from build123d import *

# Parameters (mm, degrees)
SKETCH1_W           = 66.8
SKETCH1_H           = 14
SKETCH1_R           = 1.1
BOSS_EXTRUDE2_DEPTH = 7
SKETCH5_W           = 66.8
SKETCH5_H           = 1.5
BOSS_EXTRUDE3_DEPTH = 93
SKETCH6_W           = 66.8
SKETCH6_H           = 93
SKETCH6_R           = 1
SKETCH6_W_2         = 60.8
SKETCH6_H_2         = 87
BOSS_EXTRUDE4_DEPTH = 10
FILLET1_R           = 1
CUT_EXTRUDE1_DEPTH  = 10


with BuildPart() as part:
    # Sketch1 → Boss-Extrude2 (new body)
    with BuildSketch(Plane.XY):
        Rectangle(SKETCH1_W, SKETCH1_H)
        Circle(SKETCH1_R, mode=Mode.SUBTRACT)
    extrude(amount=BOSS_EXTRUDE2_DEPTH)

    # Sketch5 → Boss-Extrude3 (add)
    with BuildSketch(Plane.XY.offset(7)):
        with Locations((0, -6.25)):
            Rectangle(SKETCH5_W, SKETCH5_H)
    extrude(amount=BOSS_EXTRUDE3_DEPTH)

    # Sketch6 → Boss-Extrude4 (add)
    with BuildSketch(Plane(origin=(0, -5.5, 0), x_dir=(1, 0, 0), z_dir=(0, 1, 0))):
        with Locations((0, -53.5)):
            Rectangle(SKETCH6_W, SKETCH6_H)
        with Locations(Location((-31.45, -8.95, 0), (0, 0, 270))):
            Circle(SKETCH6_R, mode=Mode.SUBTRACT)
        with Locations(Location((31.45, -8.95, 0), (0, 0, 270))):
            Circle(SKETCH6_R, mode=Mode.SUBTRACT)
        with Locations(Location((31.45, -98.05, 0), (0, 0, 270))):
            Circle(SKETCH6_R, mode=Mode.SUBTRACT)
        with Locations(Location((-31.45, -98.05, 0), (0, 0, 270))):
            Circle(SKETCH6_R, mode=Mode.SUBTRACT)
        with Locations((0, -53.5)):
            Rectangle(SKETCH6_W_2, SKETCH6_H_2, mode=Mode.SUBTRACT)
    extrude(amount=BOSS_EXTRUDE4_DEPTH)

    # Fillet1
    fillet1_edges = [part.edges().sort_by_distance(p)[0] for p in [
        (30.4, -0.5, 97),
        (30.4, -0.5, 10),
        (-30.4, -0.5, 10),
        (-30.4, -0.5, 97),
    ]]
    fillet(fillet1_edges, radius=FILLET1_R)

    # Sketch2 → Cut-Extrude1 (cut)
    with BuildSketch(Plane(origin=(0, 0, 0), x_dir=(-1, 0, 0), z_dir=(0, 0, -1))):
        with BuildLine():
            Line((2.7, 0), (4.75, 0))
            ThreePointArc((4.75, 0), (1.723006094, -4.426482802), (-3.5, -3.211308145))
            Line((-3.5, -3.211308145), (-1.989473684, -1.825375156))
            ThreePointArc((-1.989473684, -1.825375156), (0.979392938, -2.516106014), (2.7, 0))
        make_face()
    extrude(amount=-CUT_EXTRUDE1_DEPTH, mode=Mode.SUBTRACT)


solid = part.part
Model file for the job. Use its own axes, mm. A direction names the side the tool comes from. Give positions to 0.01 mm unless a question says otherwise; leave off trailing zeros. Order: outer loops, then holes, each group sorted by start corner. A loop starts at its lowest first (then second) coordinate and runs counter-clockwise, first axis right, second up. Notation, with made-up numbers: (19.5, -37.75) - (78.5, -37.75) arc R35 ccw to (78.5, 0.25) - close; hole circle Ø10 at (-30, -30). An arc over 180 degrees is marked (long way). Return JSON: item names as keys, results as strings.
1) Pull direction Z, two halves, no side cores. Call faces 1 (the flat face through (0, 2, 0)), 2 (the flat face through (-33.4, -2, 51)), 3 (the flat face through (0, -1, 10)): pulls with the +Z half, pulls with the -Z half, needs draft (parallel to the pull), parting line crosses it, or undercut.
Geometry says:
{"face 1": "pulls with the -Z half", "face 2": "needs draft", "face 3": "undercut"}
2) Cut at D-D, the plane z = 28.5. Give the cut face in (x, y).
Geometry says:
{"outline": "(-33.4, -7) - (33.4, -7) - (33.4, 4.5) - (30.4, 4.5) - (30.4, -5.5) - (-30.4, -5.5) - (-30.4, 4.5) - (-33.4, 4.5) - close"}
3) 3-axis set-ups, long thin cutter, end or side, ignore diameter. For faces 4 (the flat face through (31, -5.5, 98)), 5 (the flat face through (-32, 4.5, 50)), 6 (the cylindrical face through (-1.797, -4.397, 4.93)): which of +Z, -Z, +X, -X, +Y, -Y reach the whole face in a straight line?
Geometry says:
{"face 4": "+Y", "face 5": "+Z, +X, -X, +Y", "face 6": "-Z"}
4) Flat gauge pins, fed straight in: P1, Ø1.8, axis at x = 31.45, z = 98.05, coming from the +Y side; P2, Ø2, axis at x = 31.5, z = 98, coming from the +Y side; P3, Ø1.8, axis at x = 0, y = 0, coming from the -Z side. Where does each tip first touch, or does it go through?
Geometry says:
{"P1": "y = -5.5", "P2": "y = 4.5", "P3": "z = 7"}
5) Probe line 1 (X direction, y = -1.5, z = 98.05); line 2 (X direction, y = -5, z = 43); line 3 (Z direction, x = 28.5, y = -0.75). List the from-to ranges inside material, lowest first. Write a range as from..to.
Geometry says:
{"line 1": "-33.4..-32.45, -30.45..30.45, 32.45..33.4", "line 2": "-33.4..-30.4, 30.4..33.4", "line 3": "0..10, 97..100"}
6) Cut at A-A, the plane x = 0. Give the cut face in (y, z), plus the area to 3 significant figures.
Geometry says:
{"outline": "(-7, 0) - (-4.75, 0) - (-4.75, 10) - (-5.5, 10) - (-5.5, 97) - (4.5, 97) - (4.5, 100) - (-7, 100) - close; (-2.7, 0) - (-1.1, 0) - (-1.1, 7) - (1.1, 7) - (1.1, 0) - (7, 0) - (7, 7) - (4.5, 7) - (4.5, 10) - (-2.7, 10) - close", "area": "262 mm²"}
7) Cut at C-C, the plane x = -31.45. Give the cut face in (y, z), plus the area to 3 significant figures.
Geometry says:
{"outline": "(-7, 0) - (7, 0) - (7, 7) - (4.5, 7) - (4.5, 7.95) - (-5.5, 7.95) - (-5.5, 9.95) - (4.5, 9.95) - (4.5, 97.05) - (-5.5, 97.05) - (-5.5, 99.05) - (4.5, 99.05) - (4.5, 100) - (-7, 100) - close", "area": "1,130 mm²"}
8) Cut at B-B, the plane z = 8.95. Give the cut face in (x, y).
Geometry says:
{"outline": "(-33.4, -7) - (33.4, -7) - (33.4, 4.5) - (32.45, 4.5) - (32.45, -5.5) - (30.45, -5.5) - (30.45, 4.5) - (-30.45, 4.5) - (-30.45, -5.5) - (-32.45, -5.5) - (-32.45, 4.5) - (-33.4, 4.5) - close; hole (-4.75, 0) arc R4.75 ccw to (3.5, -3.21) - (1.99, -1.83) arc R2.7 cw to (-2.7, 0) - close"}
